from build123d import *

# Parameters (mm, degrees)
SKETCH1_W           = 21.413967735
SKETCH1_H           = 90
BOSS_EXTRUDE1_DEPTH = 100
CUT_EXTRUDE1_REACH  = 243.039
SKETCH2_W           = 55
SKETCH2_H           = 80
SKETCH2_W_2         = 45
SKETCH2_H_2         = 25


with BuildPart() as part:
    # Sketch1 → Boss-Extrude1 (new body)
    with BuildSketch(Plane.XY):
        with Locations((10.706983867, 45)):
            Rectangle(SKETCH1_W, SKETCH1_H)
        Polygon((200, 0), (200, 25), (21.413967735, 90), (21.413967735, 0), align=None)
    extrude(amount=BOSS_EXTRUDE1_DEPTH)

    # Cut-Extrude1: up to this face of the body (flat: up to its plane)
    cut_extrude1_end = Plane(part.part.faces().sort_by_distance((100, 0, 50))[0])
    # Sketch2 → Cut-Extrude1 (cut, up to the picked face)
    with BuildSketch(Plane(origin=(0, 90, 0), x_dir=(1, 0, 0), z_dir=(0, 1, 0)), mode=Mode.PRIVATE) as cut_extrude1_sk1:
        with Locations((48.913967735, -60)):
            Rectangle(SKETCH2_W, SKETCH2_H)
    cut_extrude1_tool1 = split(extrude(cut_extrude1_sk1.sketch, amount=-CUT_EXTRUDE1_REACH, mode=Mode.PRIVATE), bisect_by=cut_extrude1_end, keep=Keep.BOTH, mode=Mode.PRIVATE)
    # Sketch2 → Cut-Extrude1 (cut, up to the picked face)
    with BuildSketch(Plane(origin=(0, 90, 0), x_dir=(1, 0, 0), z_dir=(0, 1, 0)), mode=Mode.PRIVATE) as cut_extrude1_sk2:
        with Locations((177.5, -37.5)):
            Rectangle(SKETCH2_W_2, SKETCH2_H_2)
    cut_extrude1_tool2 = split(extrude(cut_extrude1_sk2.sketch, amount=-CUT_EXTRUDE1_REACH, mode=Mode.PRIVATE), bisect_by=cut_extrude1_end, keep=Keep.BOTH, mode=Mode.PRIVATE)
    # Sketch2 → Cut-Extrude1 (cut, up to the picked face)
    with BuildSketch(Plane(origin=(0, 90, 0), x_dir=(1, 0, 0), z_dir=(0, 1, 0)), mode=Mode.PRIVATE) as cut_extrude1_sk3:
        with Locations((177.5, -62.5)):
            Rectangle(SKETCH2_W_2, SKETCH2_H_2)
    cut_extrude1_tool3 = split(extrude(cut_extrude1_sk3.sketch, amount=-CUT_EXTRUDE1_REACH, mode=Mode.PRIVATE), bisect_by=cut_extrude1_end, keep=Keep.BOTH, mode=Mode.PRIVATE)
    add(cut_extrude1_tool1.solids().sort_by(Axis((48.913968, 90, 60), (0, -1, 0)))[0], mode=Mode.SUBTRACT)
    add(cut_extrude1_tool2.solids().sort_by(Axis((177.5, 90, 37.5), (0, -1, 0)))[0], mode=Mode.SUBTRACT)
    add(cut_extrude1_tool3.solids().sort_by(Axis((177.5, 90, 62.5), (0, -1, 0)))[0], mode=Mode.SUBTRACT)


solid = part.part
Source: CAD feature listing. Evaluate the final solid. Frame: model axes, mm. A direction names the side the tool comes from. Round coordinates to 2 decimals unless told otherwise and drop trailing zeros. Write each loop counter-clockwise with the first axis right and the second up, starting at its lowest first coordinate (ties: lowest second). Pieces come first, ordered by that corner, then holes. Notation, with made-up numbers: M 72.5,-32.5 L 90.5,-32.5 A18 cw 90.5,-14.5 Z; hole C -34.5,48.5 d10. An arc over 180 degrees is marked long. One line per item, written item: value. Start each with the question number.
Item 1: Section query D-D (y = 27). Return the cut outline in (x, z), plus the area to 3 significant figures.
Item 2: Set-up query: faces 1 (the flat face through (155, 21, 50)), 2 (the flat face through (21.414, 46, 61)), 3 (the flat face through (0, 44, 49)). Return all of +Z, -Z, +X, -X, +Y, -Y with unobstructed straight access to the full face (end or side cutting, diameter ignored); none if empty.
Item 3: Ray query, L1, parallel to X at y = 7.5, z = 46.5; L2, parallel to X at y = 84, z = 30; L3, parallel to Z at x = 63.5, y = 14. Return the intervals inside material, ascending. Write a range as from..to.
Item 4: Section query B-B (y = 18). Return the cut outline in (x, z), plus the area to 4 significant figures.
Item 5: Section query A-A (z = 86). Return the cut outline in (x, y).
Item 6: Pin query (flat end, axial travel): pin 1 (20.5 mm diameter, centred on y = 19, z = 52, fed in from +X); pin 2 (3 mm diameter, centred on x = 99, z = 85.5, fed in from +Y); pin 3 (5 mm diameter, centred on x = 144, z = 55.5, fed in from +Y). Return the tip coordinate at first contact, or that it passes through.
Item 7: Section query C-C (x = 173). Return the cut outline in (y, z).
Item 8: Mould query, pull axis Z, two halves, no side actions, for faces 4 (the flat face through (177, 16, 75)), 5 (the flat face through (49, 46, 20)), 6 (the flat face through (76.414, 35, 61)), 7 (the flat face through (76, 36, 0)). Classes: pulls with the +Z half, pulls with the -Z half, needs draft (parallel to the pull), parting line crosses it, or undercut.
Result set:
1. outline: M 0,0 L 194.51,0 L 194.51,25 L 155,25 L 155,75 L 194.51,75 L 194.51,100 L 76.41,100 L 76.41,20 L 21.41,20 L 21.41,100 L 0,100 Z
1. area: 13,100 mm²
2. face 1: +X, +Y, -Y
2. face 2: +Z, +Y, -Y
2. face 3: +Z, -Z, -X, +Y, -Y
3. L1: x = 0..21.41, 76.41..155
3. L2: x = 0..21.41
3. L3: z = 0..20
4. outline: M 0,0 L 200,0 L 200,25 L 155,25 L 155,75 L 200,75 L 200,100 L 76.41,100 L 76.41,20 L 21.41,20 L 21.41,100 L 0,100 Z
4. area: 13,350 mm²
5. outline: M 0,0 L 21.41,0 L 21.41,90 L 0,90 Z; M 76.41,0 L 200,0 L 200,25 L 76.41,69.98 Z
6. pin 1: stops at x = 155
6. pin 2: stops at y = 62.31
6. pin 3: stops at y = 46.29
7. outline: M 0,0 L 34.83,0 L 34.83,25 L 0,25 Z; M 0,75 L 34.83,75 L 34.83,100 L 0,100 Z
8. face 4: undercut
8. face 5: pulls with the +Z half
8. face 6: needs draft
8. face 7: pulls with the -Z half
